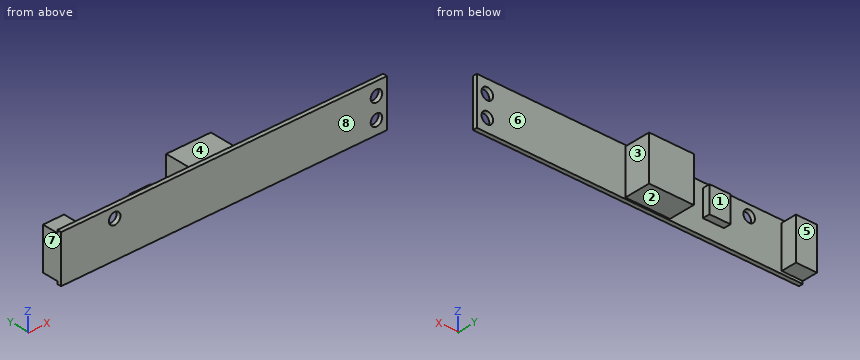
```python
from build123d import *

# Parameters (mm, degrees)
SKETCH_1_W      = 62
SKETCH_1_H      = 9
SKETCH_1_R      = 1.1
EXTRUDE_1_DEPTH = 0.8
SKETCH_3_W      = 8.5
SKETCH_3_H      = 8.5
EXTRUDE_2_DEPTH = 5
EXTRUDE_3_DEPTH = 3
SKETCH_5_W      = 4
SKETCH_5_H      = 5
EXTRUDE_4_DEPTH = 1.4


with BuildPart() as part:
    # 草图1 → 凸台-拉伸1 (new body)
    with BuildSketch(Plane(origin=(0, 0, 0), x_dir=(1, 0, 0), z_dir=(0, 1, 0))):
        Rectangle(SKETCH_1_W, SKETCH_1_H)
        with Locations(Location((29, 2, 0), (0, 0, 270))):
            Circle(SKETCH_1_R, mode=Mode.SUBTRACT)
        with Locations(Location((29, -2, 0), (0, 0, 90))):
            Circle(SKETCH_1_R, mode=Mode.SUBTRACT)
        with Locations(Location((-20.8, -2.5, 0), (0, 0, 270))):
            Circle(SKETCH_1_R, mode=Mode.SUBTRACT)
    extrude(amount=EXTRUDE_1_DEPTH)

    # 草图3 → 凸台-拉伸2 (add)
    with BuildSketch(Plane(origin=(0, 0.8, 0), x_dir=(1, 0, 0), z_dir=(0, 1, 0))):
        with Locations((-1.5, 0)):
            Rectangle(SKETCH_3_W, SKETCH_3_H)
    extrude(amount=EXTRUDE_2_DEPTH)

    # 草图4 → 凸台-拉伸3 (add)
    with BuildSketch(Plane(origin=(0, 0.8, 0), x_dir=(1, 0, 0), z_dir=(0, 1, 0))):
        Polygon((-31, 0), (-31, 4), (-27, 4), (-27, -1.222216668), (-27, -4), (-31, -4), align=None)
    extrude(amount=EXTRUDE_3_DEPTH)

    # 草图5 → 凸台-拉伸4 (add)
    with BuildSketch(Plane(origin=(0, 0.8, 0), x_dir=(1, 0, 0), z_dir=(0, 1, 0))):
        with Locations((-14, -1)):
            Rectangle(SKETCH_5_W, SKETCH_5_H)
    extrude(amount=EXTRUDE_4_DEPTH)


solid = part.part
```
Build history of the part. All positions in model axes, mm. Face numbers are marked on the shaded views. A direction names the side the tool comes from. Round coordinates to 2 decimals unless told otherwise and drop trailing zeros. Loops run counter-clockwise (first coordinate to the right, second up) from the corner with the lowest first, then second, coordinate; pieces in that order, holes last. Notation, with made-up numbers: M -3,-7.5 L 31,-7.5 A12 ccw 31,11.5 Z; hole C 87,54.5 d3. An arc over 180 degrees is marked long. Answer as CSV lines item,"result".
1. Cut at C-C on x = 29. Write the cut outline in (y, z).
Resolved:
outline,"M 0,-4.5 L 0.8,-4.5 L 0.8,-3.1 L 0,-3.1 Z; M 0,-0.9 L 0.8,-0.9 L 0.8,0.9 L 0,0.9 Z; M 0,3.1 L 0.8,3.1 L 0.8,4.5 L 0,4.5 Z"
2. Cut at B-B on z = 2. Write the cut outline in (x, y), then the cut area to 3 significant figures.
Resolved:
outline,"M -31,0 L -21.78,0 L -21.78,0.8 L -27,0.8 L -27,3.8 L -31,3.8 Z; M -19.82,0 L 27.9,0 L 27.9,0.8 L 2.75,0.8 L 2.75,5.8 L -5.75,5.8 L -5.75,0.8 L -12,0.8 L -12,2.2 L -16,2.2 L -16,0.8 L -19.82,0.8 Z; M 30.1,0 L 31,0 L 31,0.8 L 30.1,0.8 Z"
area,"106 mm²"
3. Flat gauge pins, fed straight in: P1, Ø1.5, axis at y = 1.5, z = 2, coming from the +X side; P2, Ø3, axis at x = -29.5, z = 1.5, coming from the +Y side; P3, Ø3, axis at x = -14.5, z = 1.5, coming from the +Y side; P4, Ø1.5, axis at x = -28, y = 3, coming from the -Z side. Where does each tip first touch, or does it go through?
Resolved:
P1,"stops at x = 31"
P2,"stops at y = 3.8"
P3,"stops at y = 2.2"
P4,"stops at z = -4"
4. Cut at A-A on x = -20.8. Write the cut outline in (y, z), then the cut area to 3 significant figures.
Resolved:
outline,"M 0,-4.5 L 0.8,-4.5 L 0.8,1.4 L 0,1.4 Z; M 0,3.6 L 0.8,3.6 L 0.8,4.5 L 0,4.5 Z"
area,"5.44 mm²"
5. Wall check: probe 1 along X at (y, z) = (0.25, -2); probe 2 along X at (y, z) = (3.35, 0); probe 3 along X at (y, z) = (0.4, 2). Give the ranges that are in metal, low to high. Write a range as [from, to].
Resolved:
probe 1,"x = [-31, 27.9], [30.1, 31]"
probe 2,"x = [-31, -27], [-5.75, 2.75]"
probe 3,"x = [-31, -21.78], [-19.82, 27.9], [30.1, 31]"
6. 3-axis set-ups, long thin cutter, end or side, ignore diameter. For the marked faces 1, 2, 3, 4 and 5: which of +Z, -Z, +X, -X, +Y, -Y reach the whole face in a straight line?
Resolved:
face 1,"+Z, -Z, +Y"
face 2,"-Z, +X, -X, +Y"
face 3,"+Z, -Z, +X, +Y"
face 4,"+Z, +X, -X, +Y"
face 5,"+Z, -Z, -X, +Y"
7. Cut at D-D on x = -14. Write the cut outline in (y, z), then the cut area to 3 significant figures.
Resolved:
outline,"M 0,-4.5 L 0.8,-4.5 L 0.8,-1.5 L 2.2,-1.5 L 2.2,3.5 L 0.8,3.5 L 0.8,4.5 L 0,4.5 Z"
area,"14.2 mm²"
8. Two-plate mould, pull along X, no slides. Class the marked faces 6, 7 and 8: released by +X, released by -X, zero draft, split by the parting line, or undercut.
Resolved:
face 6,"undercut"
face 7,"released by -X"
face 8,"zero draft"
